The model under review builds one solid part; all positions refer to its coordinate system, in mm. Face numbers are marked on the shaded views. A direction names the side the tool comes from. Round coordinates to 2 decimals unless told otherwise and drop trailing zeros. Write each loop counter-clockwise with the first axis right and the second up, starting at its lowest first coordinate (ties: lowest second). Pieces come first, ordered by that corner, then holes. Notation, with made-up numbers: (38.25, 72) - (49.25, 72) arc R33 ccw to (49.25, 109) - close; hole circle Ø7 at (-21.75, 17.5). An arc over 180 degrees is marked (long way). One line per question, with ' | ' between items. Start each with the question number.
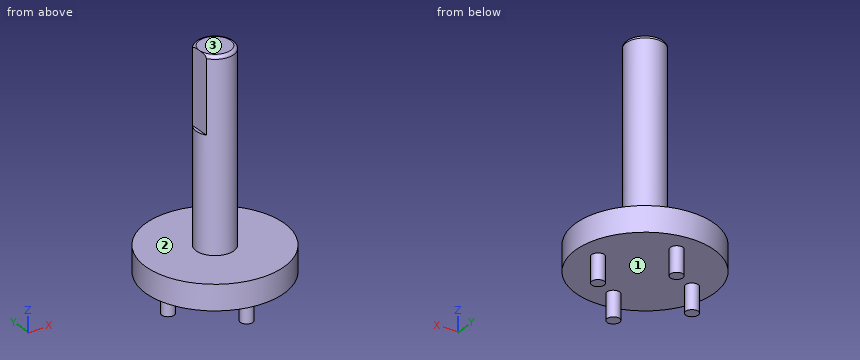
Autodesk Inventor part; units mm, degrees
ref_plane "YZ Plane" through (0, 0, 0) normal (1, 0, 0) x (0, 1, 0)
ref_plane "XZ Plane" through (0, 0, 0) normal (0, 1, 0) x (-1, 0, 0)
ref_plane "XY Plane" through (0, 0, 0) normal (0, 0, 1) x (1, 0, 0)
sketch "スケッチ1" plane through (0, 0, 0) normal (0, 0, 1) x (1, 0, 0)
  circle A0 centre (0, 0) radius 11
  dimension "d0" = 22
extrude "押し出し1" add sketch "スケッチ1" along normal blind 4
sketch "スケッチ2" plane through (0, 0, 4) normal (0, 0, 1) x (1, 0, 0)
  circle A0 centre (0, 0) radius 11
  circle A1 centre (0, 0) radius 3
  dimension "d3" = 6
extrude "押し出し2" add sketch "スケッチ2" along normal blind 30 contours A1
sketch "スケッチ3" plane through (0, 0, 0) normal (0, 0, -1) x (-1, 0, 0)
  circle A0 centre (0, 7.5) radius 1
  circle A1 centre (-7.5, 0) radius 1
  circle A2 centre (0, -7.5) radius 1
  circle A3 centre (7.5, 0) radius 1
  point P0 (0, 0)
  dimension "d6" = 2
  dimension "d7" = 7.5
  dimension "d10" = 360
extrude "押し出し3" add sketch "スケッチ3" along normal blind 4
fillet "フィレット1" radius 0.5 1 edges at (-3, 0, 34)
sketch "スケッチ4" plane through (0, 0, 34) normal (0, 0, 1) x (1, 0, 0)
  line L0 (-3, -1.6583) -> (-2.5, -1.6583)
  line L1 (-2.5, -1.6583) -> (-2.5, 1.6583)
  line L2 (-2.5, 1.6583) -> (-3, 1.6583)
  line L3 (-3, 1.6583) -> (-3, -1.6583)
  circle A0 centre (0, 0) radius 3
  point P0 (-2.5, 0)
  dimension "d15" = 0.5
extrude "押し出し4" cut sketch "スケッチ4" against normal blind 12 contours A0 L1 picked at (-2.5914, 0.3806)
properties part number "555_GearBox_Shaft" material "鉄、鋳鉄"
1. Add section D-D, the plane x = -4.75. Write out the cut boundary in (y, z), then the cut area to 3 significant figures.
2. Add section A-A, the plane y = 7.5. Write out the cut boundary in (x, z).
3. Machinability: for the marked faces 1, 2 and 3, which of the approach directions +Z, -Z, +X, -X, +Y, -Y give a long, thin tool a straight path to every point of the face, cutting with its end or side? Answer none if there is none.
4. Wall thickness on line 1 along Z through (x, y) = (9.5, 5.25); line 2 along Z through (x, y) = (-0.75, 8); line 3 along Y through (x, z) = (1.25, 15): over which ranges is each line inside the solid? List them lowest first. Write a range as [from, to].
5. Add section C-C, the plane z = 30. Write out the cut boundary in (x, y), then the cut area to 3 significant figures.
6. Clearance check with flat-ended pins moving along their axes: P1, Ø8, axis at y = 0.5, z = 2, coming from the +X side; P2, Ø1, axis at x = 6.5, y = -2, coming from the -Z side; P3, Ø5, axis at y = 1.5, z = 20, coming from the +X side; P4, Ø8, axis at y = -4.5, z = 14.5, coming from the -X side. State where each tip first meets the part, or that it passes through.
Geometry check:
1) outline: (-9.92, 0) - (9.92, 0) - (9.92, 4) - (-9.92, 4) - close | area: 79.4 mm2
2) outline: (-8.05, 0) - (-1, 0) - (-1, -4) - (1, -4) - (1, 0) - (8.05, 0) - (8.05, 4) - (-8.05, 4) - close
3) face 1: -Z | face 2: +Z | face 3: +Z, +X, -X, +Y, -Y
4) line 1: z = [0, 4] | line 2: z = [-4, 4] | line 3: y = [-2.73, 2.73]
5) outline: (-2.5, -1.66) arc R3 ccw (long way) to (-2.5, 1.66) - close | area: 27.1 mm2
6) P1: stops at x = 11 | P2: stops at z = 0 | P3: stops at x = 3 | P4: stops at x = -2.96
